The model under review builds one solid part; all positions refer to its coordinate system, in mm. Coordinates: 2 decimals unless noted, no trailing zeros. Loops run counter-clockwise (first coordinate to the right, second up) from the corner with the lowest first, then second, coordinate; pieces in that order, holes last. Notation, with made-up numbers: M -4,-12.5 L 38,-12.5 A25 cw 38,25.5 Z; hole C 15.25,55.5 d1. An arc over 180 degrees is marked long. Use CSV: the item, a comma, the result in double quotes. Start each with the question number.
1. For L1, parallel to X at y = 8, z = -8.75; L2, parallel to Y at x = -1, z = -6; L3, parallel to X at y = 0, z = -13.5, list the stretches that pass through material, from the lowest coordinate up.
2. Add section D-D, the plane y = 23.5. Write out the cut boundary in (x, z), then the cut area to 3 significant figures.
3. Add section C-C, the plane x = 13. Write out the cut boundary in (y, z), then the cut area to 3 significant figures.
4. Draft analysis for pull direction X (two halves, no side actions). For faces 1 (the flat face through (-15.19, 11.43, -9.02)), 2 (the cylindrical face through (2.87, 11.07, -9.02)), 3 (the flat face through (19.34, 7.26, -9.02)), state which applies: +X half, -X half, draft (parallel to the pull), parting line (faces both ways), or undercut.
5. Add section B-B, the plane z = -15.25. Write out the cut boundary in (x, y), then the cut area to 3 significant figures.
6. Clearance check with flat-ended pins moving along their axes: P1, Ø1.5, axis at y = -6, z = -8.5, coming from the +X side; P2, Ø1.5, axis at y = 5, z = -5, coming from the +X side; P3, Ø1, axis at y = -4.5, z = -14.5, coming from the +X side. State where each tip first meets the part, or that it passes through.
7. Add section A-A, the plane y = 4.5. Write out the cut boundary in (x, z), then the cut area to 3 significant figures.
from build123d import *

# Parameters (mm, degrees)
F1_DEPTH = 18.288
F3_D     = 7.62


with BuildPart() as f1:
    # F0 (on Top) → F1 (new body)
    with BuildSketch(Plane.XY):
        Polygon((-16.326535, 1.318186), (-0.170244, -10.602742), (18.231728, -2.571448), (20.477409, 17.380775), (4.321118, 29.301702), (-14.080854, 21.270408), align=None)
    extrude(amount=-F1_DEPTH)

    # F3 (through all)
    with Locations(Plane(origin=(0, 0, -18.288), x_dir=(1, 0, 0), z_dir=(0, 0, -1))):
        with Locations((2.046527, -7.350766)):
            Hole(F3_D / 2)


solid = f1.part
Computed:
1,L1,"x = -15.57 to -1.71, 5.8 to 19.42"
1,L2,"y = -9.99 to 5.06, 9.64 to 26.98"
1,L3,"x = -14.54 to 18.52"
2,outline,"M -8.97,-18.29 L 12.18,-18.29 L 12.18,0 L -8.97,0 Z"
2,area,"387 mm^2"
3,outline,"M -4.85,-18.29 L 22.9,-18.29 L 22.9,0 L -4.85,0 Z"
3,area,"508 mm^2"
4,face 1,"-X half"
4,face 2,"undercut"
4,face 3,"+X half"
5,outline,"M -16.33,1.32 L -0.17,-10.6 L 18.23,-2.57 L 20.48,17.38 L 4.32,29.3 L -14.08,21.27 Z; hole C 2.05,7.35 d7.62"
5,area,"1,000 mm^2"
6,P1,"stops at x = 12.09"
6,P2,"stops at x = 19.17"
6,P3,"stops at x = 14.96"
7,outline,"M -15.97,-18.29 L -0.48,-18.29 L -0.48,0 L -15.97,0 Z; M 4.57,-18.29 L 19.03,-18.29 L 19.03,0 L 4.57,0 Z"
7,area,"548 mm^2"
